```python
from build123d import *

# Parameters (mm, degrees)
F0_W           = 90
F0_H           = 110
F1_DEPTH       = 19
F2_W           = 50
F2_H           = 110
F3_DEPTH       = 4
F5_D           = 11
F5_CBORE_D     = 17.25
F5_CBORE_DEPTH = 10
F8_D           = 6.8
F8_DEPTH       = 23.75
F8_TIP         = 2.0429261047
F8_ON_F7_D     = 6.8
F8_ON_F7_DEPTH = 23.75
F8_ON_F7_TIP   = 2.0429261047
F9_SIZE        = 0.5


with BuildPart() as f1:
    # F0 (on Front) → F1 (new body)
    with BuildSketch(Plane.XZ):
        with Locations((-45, 55)):
            Rectangle(F0_W, F0_H)
    extrude(amount=F1_DEPTH)

    # F2 (on face) → F3 (cut)
    with BuildSketch(Plane.XZ.offset(19)):
        with Locations((-45, 55)):
            Rectangle(F2_W, F2_H)
    extrude(amount=-F3_DEPTH, mode=Mode.SUBTRACT)

    # F5 (through all)
    with Locations(Plane(origin=(0, 0, 0), x_dir=(-1, 0, 0), z_dir=(0, 1, 0))):
        with Locations((45, 72), (45, 44), (45, 16)):
            CounterBoreHole(F5_D / 2, F5_CBORE_D / 2, F5_CBORE_DEPTH)

    # F8
    with Locations(Plane.YZ):
        with Locations((-9.5, 90), (-9.5, 20)):
            Hole(F8_D / 2, depth=F8_DEPTH)
            with Locations((0, 0, -(F8_DEPTH + F8_TIP / 2))):  # 118° drill point
                Cone(0, F8_D / 2, F8_TIP, mode=Mode.SUBTRACT)

    # F8 on F7
    with Locations(Plane(origin=(-90, 0, 0), x_dir=(0, -1, 0), z_dir=(-1, 0, 0))):
        with Locations((9.5, 90), (9.5, 20)):
            Hole(F8_ON_F7_D / 2, depth=F8_ON_F7_DEPTH)
            with Locations((0, 0, -(F8_ON_F7_DEPTH + F8_ON_F7_TIP / 2))):  # 118° drill point
                Cone(0, F8_ON_F7_D / 2, F8_ON_F7_TIP, mode=Mode.SUBTRACT)

    # F9
    f9_edges = [f1.edges().sort_by_distance(p)[0] for p in [
        (-45, 0, 110),
        (-90, -9.5, 110),
        (-80, -19, 110),
        (-70, -17, 110),
        (-45, -15, 110),
        (-20, -17, 110),
        (-10, -19, 110),
        (0, -9.5, 110),
        (-45, 0, 0),
        (0, -9.5, 0),
        (-10, -19, 0),
        (-20, -17, 0),
        (-45, -15, 0),
        (-70, -17, 0),
        (-80, -19, 0),
        (-90, -9.5, 0),
        (0, 0, 55),
        (0, -19, 55),
        (0, -12.9, 20),
        (0, -12.9, 90),
        (-90, 0, 55),
        (-90, -19, 55),
        (-90, -6.1, 90),
        (-90, -6.1, 20),
        (-36.375, 0, 16),
        (-36.375, 0, 44),
        (-36.375, 0, 72),
    ]]
    chamfer(f9_edges, length=F9_SIZE)


solid = f1.part
```
The model under review builds one solid part; all positions refer to its coordinate system, in mm. A direction names the side the tool comes from. Round coordinates to 2 decimals unless told otherwise and drop trailing zeros. Order: outer loops, then holes, each group sorted by start corner. A loop starts at its lowest first (then second) coordinate and runs counter-clockwise, first axis right, second up. Notation, with made-up numbers: (7, 84.25) -> (26, 84.25) arc R21 cw to (26, 90.25) -> close; hole circle Ø6 at (50, 66.25). An arc over 180 degrees is marked (long way). Use a Markdown table: item, result.
Q1. Mouldability with a two-part tool opening along X and no side actions: class faces 5 (the flat face through (-46, -9, 0)), 6 (the flat face through (-90, -9, 54)), 7 (the cylindrical face through (-52.97, -5.18, 12.7)), 8 (the flat face through (-70, -17, 54)) as +X half, -X half, draft (parallel to the pull), parting line (faces both ways), or undercut.
Values:
| item | result |
|---|---|
| face 5 | draft |
| face 6 | -X half |
| face 7 | undercut |
| face 8 | undercut |
Q2. We need section B-B on x = -22.5. Write out the cut boundary in (y, z), then the cut area to 3 significant figures.
Values:
| item | result |
|---|---|
| outline | (-15, 0.5) -> (-14.5, 0) -> (-0.5, 0) -> (0, 0.5) -> (0, 109.5) -> (-0.5, 110) -> (-14.5, 110) -> (-15, 109.5) -> close; hole circle Ø6.8 at (-9.5, 20); hole circle Ø6.8 at (-9.5, 90) |
| area | 1,580 mm^2 |
Q3. Tool access review of faces 1 (the cylindrical face through (-12.29, -8.76, 86.68)), 2 (the flat face through (-10, -19, 56)), 3 (the flat face through (-51, -10, 72)), 4 (the cylindrical face through (-77.7, -7.9, 17)): name each direction out of +Z, -Z, +X, -X, +Y, -Y from which nothing blocks a thin tool from reaching the whole face with its end or side.
Values:
| item | result |
|---|---|
| face 1 | +X |
| face 2 | +Z, -Z, +X, -X, -Y |
| face 3 | +Y |
| face 4 | -X |
Q4. For line 1 (Z direction, x = -16, y = -9.5); line 2 (X direction, y = -15.5, z = 103.5); line 3 (Y direction, x = -80, z = 20), list the stretches that pass through material, from the lowest coordinate up.
Values:
| item | result |
|---|---|
| line 1 | z = 0 to 16.6, 23.4 to 86.6, 93.4 to 110 |
| line 2 | x = -90 to -70, -20 to 0 |
| line 3 | y = -19 to -12.9, -6.1 to 0 |
Q5. We need section A-A on z = 72. Write out the cut boundary in (x, y) (3 decimals), then the cut area to 3 significant figures.
Values:
| item | result |
|---|---|
| outline | (-90, -18.5) -> (-89.5, -19) -> (-70, -19) -> (-70, -15) -> (-50.5, -15) -> (-50.5, -10) -> (-53.625, -10) -> (-53.625, -0.5) -> (-54.125, 0) -> (-89.5, 0) -> (-90, -0.5) -> close; (-39.5, -15) -> (-20, -15) -> (-20, -19) -> (-0.5, -19) -> (0, -18.5) -> (0, -0.5) -> (-0.5, 0) -> (-35.875, 0) -> (-36.375, -0.5) -> (-36.375, -10) -> (-39.5, -10) -> close |
| area | 1,280 mm^2 |
Q6. Clearance check with flat-ended pins moving along their axes: P1, Ø1.5, axis at y = -9.5, z = 23.5, coming from the +X side; P2, Ø6, axis at x = -25, z = 41.5, coming from the -Y side; P3, Ø4, axis at y = -9.5, z = 20, coming from the -X side; P4, Ø8.5, axis at x = -48, z = 12.5, coming from the +Y side. State where each tip first meets the part, or that it passes through.
Values:
| item | result |
|---|---|
| P1 | stops at x = 0 |
| P2 | stops at y = -15 |
| P3 | stops at x = -65.41 |
| P4 | stops at y = -0.27 |
Q7. We need section C-C on y = -17.25. Write out the cut boundary in (x, z).
Values:
| item | result |
|---|---|
| outline | (-90, 0.5) -> (-89.5, 0) -> (-70.5, 0) -> (-70, 0.5) -> (-70, 109.5) -> (-70.5, 110) -> (-89.5, 110) -> (-90, 109.5) -> close; (-20, 0.5) -> (-19.5, 0) -> (-0.5, 0) -> (0, 0.5) -> (0, 109.5) -> (-0.5, 110) -> (-19.5, 110) -> (-20, 109.5) -> close |
Q8. We need section D-D on y = -2.25. Write out the cut boundary in (x, z) (3 decimals), then the cut area to 3 significant figures.
Values:
| item | result |
|---|---|
| outline | (-90, 0.5) -> (-89.5, 0) -> (-0.5, 0) -> (0, 0.5) -> (0, 109.5) -> (-0.5, 110) -> (-89.5, 110) -> (-90, 109.5) -> close; hole circle Ø17.25 at (-45, 16); hole circle Ø17.25 at (-45, 44); hole circle Ø17.25 at (-45, 72) |
| area | 9,200 mm^2 |
